For this review, take the finished solid that the model builds, in its own axes (mm). A direction names the side the tool comes from. Give positions to 0.01 mm unless a question says otherwise; leave off trailing zeros. Order: outer loops, then holes, each group sorted by start corner. A loop starts at its lowest first (then second) coordinate and runs counter-clockwise, first axis right, second up.
Item 1: The part is to be moulded in two halves that separate along X. For faces 1 (the flat face through (1, -8, 69)), 2 (the flat face through (-71, -22.48, -25)), 3 (the flat face through (75, -9, 1)), say which applies: released by +X, released by -X, zero draft, split by the parting line, or undercut.
Item 2: Consider section A-A (z = 47.5). Give the boundary of the cut face in (x, y), plus the area to 3 significant figures.
Item 3: Consider section B-B (x = 25). Give the boundary of the cut face in (y, z), plus the area to 3 significant figures.
Item 4: Machinability: for faces 4 (the flat face through (-25, -22.48, -71)), 5 (the cylindrical face through (73.063, -19.945, 25.751)), 6 (the flat face through (-38, -8, 74)), which of the approach directions +Z, -Z, +X, -X, +Y, -Y give a long, thin tool a straight path to every point of the face, cutting with its end or side? Answer none if there is none.
Item 5: Consider section C-C (y = -19.5). Give the boundary of the cut face in (x, z), plus the area to 3 significant figures.
Item 6: For probe 1 along Z at (x, y) = (-13.5, -6); probe 2 along Y at (x, z) = (1, 68), list the stretches that pass through material, from the lowest coordinate up.
Item 7: Consider section D-D (y = -1.75). Give the boundary of the cut face in (x, z).
```python
from build123d import *

# Parameters (mm, degrees)
SKETCH1_W           = 150
SKETCH1_H           = 150
BOSS_EXTRUDE1_DEPTH = 17.48
SKETCH2_W           = 148
SKETCH2_H           = 148
CUT_EXTRUDE1_DEPTH  = 16.48
SKETCH3_W           = 132
SKETCH3_H           = 132
CUT_EXTRUDE2_DEPTH  = 2
SKETCH4_W           = 5
SKETCH4_H           = 17.47
BOSS_EXTRUDE3_DEPTH = 5
CIRPATTERN2_COUNT   = 4
SKETCH6_R           = 2.5
BOSS_EXTRUDE5_DEPTH = 5


with BuildPart() as part:
    # Sketch1 → Boss-Extrude1 (new body)
    with BuildSketch(Plane(origin=(0, 0, 0), x_dir=(1, 0, 0), z_dir=(0, 1, 0))):
        Rectangle(SKETCH1_W, SKETCH1_H)
    extrude(amount=-BOSS_EXTRUDE1_DEPTH)

    # Sketch2 → Cut-Extrude1 (cut)
    with BuildSketch(Plane(origin=(0, 0, 0), x_dir=(1, 0, 0), z_dir=(0, 1, 0))):
        Rectangle(SKETCH2_W, SKETCH2_H)
    extrude(amount=-CUT_EXTRUDE1_DEPTH, mode=Mode.SUBTRACT)

    # Sketch3 → Cut-Extrude2 (cut, through all)
    with BuildSketch(Plane(origin=(0, -16.48, 0), x_dir=(1, 0, 0), z_dir=(0, 1, 0))):
        Rectangle(SKETCH3_W, SKETCH3_H)
    extrude(amount=-CUT_EXTRUDE2_DEPTH, mode=Mode.SUBTRACT)

    # Sketch4 → Boss-Extrude3 (add)
    with BuildSketch(Plane.XY.offset(-74)):
        with Locations((-1, -8.735)):
            Rectangle(SKETCH4_W, SKETCH4_H)
    boss_extrude3 = extrude(amount=BOSS_EXTRUDE3_DEPTH)

    # CirPattern2: Boss-Extrude3 ×4 about axis
    cirpattern2_axis = Axis((0, 0, 0), (0, 1, 0))
    for i in range(1, CIRPATTERN2_COUNT):
        add(boss_extrude3.rotate(cirpattern2_axis, i * 360 / CIRPATTERN2_COUNT))

    # Sketch6 → Boss-Extrude5 (add)
    with BuildSketch(Plane.XZ.offset(17.48)):
        with Locations((-70.678187872, -25)):
            Circle(SKETCH6_R)
        with Locations((-70.678187872, 25)):
            Circle(SKETCH6_R)
        with Locations((25, 70.678187872)):
            Circle(SKETCH6_R)
        with Locations((-25, 70.678187872)):
            Circle(SKETCH6_R)
        with Locations((70.678187872, -25)):
            Circle(SKETCH6_R)
        with Locations((70.678187872, 25)):
            Circle(SKETCH6_R)
        with Locations((-25, -70.678187872)):
            Circle(SKETCH6_R)
        with Locations((25, -70.678187872)):
            Circle(SKETCH6_R)
    extrude(amount=BOSS_EXTRUDE5_DEPTH)


solid = part.part
```
Resolved:
1. face 1: undercut
1. face 2: zero draft
1. face 3: released by +X
2. outline: (-75, -17.48) - (-66, -17.48) - (-66, -16.48) - (-74, -16.48) - (-74, 0) - (-75, 0) - close; (66, -17.48) - (75, -17.48) - (75, 0) - (74, 0) - (74, -16.48) - (66, -16.48) - close
2. area: 51.0 mm2
3. outline: (-22.48, -73.18) - (-17.48, -73.18) - (-17.48, -75) - (0, -75) - (0, -74) - (-16.48, -74) - (-16.48, -66) - (-17.48, -66) - (-17.48, -68.18) - (-22.48, -68.18) - close; (-22.48, 68.18) - (-17.48, 68.18) - (-17.48, 66) - (-16.48, 66) - (-16.48, 74) - (0, 74) - (0, 75) - (-17.48, 75) - (-17.48, 73.18) - (-22.48, 73.18) - close
3. area: 101 mm2
4. face 4: +Z, -Z, +X, -X, -Y
4. face 5: -Y
4. face 6: +Y
5. outline: circle Ø5 at (-70.68, -25); circle Ø5 at (-70.68, 25); circle Ø5 at (-25, -70.68); circle Ø5 at (-25, 70.68); circle Ø5 at (25, -70.68); circle Ø5 at (25, 70.68); circle Ø5 at (70.68, -25); circle Ø5 at (70.68, 25)
5. area: 157 mm2
6. probe 1: z = -75 to -74, 74 to 75
6. probe 2: y = -17.48 to -16.48
7. outline: (-75, -75) - (75, -75) - (75, 75) - (-75, 75) - close; hole (-74, -74) - (-3.5, -74) - (-3.5, -69) - (1.5, -69) - (1.5, -74) - (74, -74) - (74, -3.5) - (69, -3.5) - (69, 1.5) - (74, 1.5) - (74, 74) - (3.5, 74) - (3.5, 69) - (-1.5, 69) - (-1.5, 74) - (-74, 74) - (-74, 3.5) - (-69, 3.5) - (-69, -1.5) - (-74, -1.5) - close
